The model under review builds one solid part; all positions refer to its coordinate system, in mm. A direction names the side the tool comes from. Round coordinates to 2 decimals unless told otherwise and drop trailing zeros. Order: outer loops, then holes, each group sorted by start corner. A loop starts at its lowest first (then second) coordinate and runs counter-clockwise, first axis right, second up. Notation, with made-up numbers: M 43,75 L 66,75 A11 ccw 66,86 Z; hole C 87,19.5 d6. An arc over 180 degrees is marked long. Answer as CSV lines item,"result". Start each with the question number.
from build123d import *

# Parameters (mm, degrees)
BOSS_EXTRUDE1_DEPTH = 12.7
SKETCH2_R           = 3.499999985
CUT_EXTRUDE1_DEPTH  = 127


with BuildPart() as part:
    # Sketch1 → Boss-Extrude1 (new body)
    with BuildSketch(Plane.XY):
        with BuildLine():
            Line((-3.110307402, -37.00399852), (-3.110307402, -54.746228005))
            Line((-3.110307402, -54.746228005), (-7.465236153, -54.746228005))
            Line((-7.465236153, -54.746228005), (-7.465236153, -42.046228005))
            ThreePointArc((-7.465236153, -42.046228005), (-12.933427118, -37.502447849), (-15.956082844, -31.067340787))
            ThreePointArc((-15.956082844, -31.067340787), (-18.522349701, -15.547297089), (-18.849139709, 0.180089543))
            ThreePointArc((-18.849139709, 0.180089543), (0, 18.85), (18.849139709, 0.180089543))
            ThreePointArc((18.849139709, 0.180089543), (18.522349701, -15.547297089), (15.956082844, -31.067340787))
            ThreePointArc((15.956082844, -31.067340787), (12.933427118, -37.502447849), (7.465236153, -42.046228005))
            Line((7.465236153, -42.046228005), (7.465236153, -54.746228005))
            Line((7.465236153, -54.746228005), (3.110307402, -54.746228005))
            Line((3.110307402, -54.746228005), (3.110307402, -37.00399852))
            ThreePointArc((3.110307402, -37.00399852), (7.417993382, -34.206219068), (9.768536138, -29.639088993))
            ThreePointArc((9.768536138, -29.639088993), (12.203438759, -14.918076577), (12.5, 0))
            ThreePointArc((12.5, 0), (0, 12.5), (-12.5, 0))
            ThreePointArc((-12.5, 0), (-12.203438759, -14.918076577), (-9.768536138, -29.639088993))
            ThreePointArc((-9.768536138, -29.639088993), (-7.417993382, -34.206219068), (-3.110307402, -37.00399852))
        make_face()
    extrude(amount=BOSS_EXTRUDE1_DEPTH)

    # Sketch2 → Cut-Extrude1 (cut)
    with BuildSketch(Plane(origin=(7.465236153, 0, 0), x_dir=(0, 0, -1), z_dir=(1, 0, 0))):
        with Locations(Location((-6.35, -48.396228005, 0), (0, 0, 90))):
            Circle(SKETCH2_R)
    extrude(amount=-CUT_EXTRUDE1_DEPTH, mode=Mode.SUBTRACT)


solid = part.part
Item 1: Tool access review of faces 1 (the flat face through (-7.465, -46, 3)), 2 (the cylindrical face through (0.275, 12.497, 6.261)), 3 (the flat face through (7.465, -45, 9)), 4 (the cylindrical face through (-5.257, -51.893, 6.504)), 5 (the flat face through (3.11, -44, 6)): name each direction out of +Z, -Z, +X, -X, +Y, -Y from which nothing blocks a thin tool from reaching the whole face with its end or side.
Item 2: Consider section B-B (y = -4.5). State the section outline as (x, z) points.
Item 3: For pin 1 (1 mm diameter, centred on y = 10, z = 4, fed in from +X); pin 2 (4 mm diameter, centred on y = -46, z = 3.5, fed in from -X); pin 3 (6.5 mm diameter, centred on y = -50, z = 5.5, fed in from +X); pin 4 (12 mm diameter, centred on x = -13.5, y = -32.5, fed in from -Z), all flat-tipped, find the tip position at first contact; note any pin that passes through.
Item 4: Wall thickness on probe 1 along X at (y, z) = (-5, 0.5); probe 2 along Y at (x, z) = (4, 8.25); probe 3 along Z at (x, y) = (7, -48.5): over which ranges is each line inside the solid? List them lowest first. Write a range as [from, to].
Item 5: The part is to be moulded in two halves that separate along X. For faces 6 (the flat face through (-5, -54.746, 6)), 7 (the cylindrical face through (18.542, -15.328, 6.261)), 8 (the cylindrical face through (12.184, -15.126, 6.261)), say which applies: +X half, -X half, draft (parallel to the pull), parting line (faces both ways), or undercut.
Item 6: Consider section D-D (x = -0.5). State the section outline as (y, z) points, and give its area (3 significant figures).
Reported:
1,face 1,"+Z, -Z, -X, -Y"
1,face 2,"+Z, -Z"
1,face 3,"+Z, -Z, +X, -Y"
1,face 4,"+X, -X"
1,face 5,"+Z, -Z, -Y"
2,outline,"M -18.99,0 L -12.64,0 L -12.64,12.7 L -18.99,12.7 Z; M 12.64,0 L 18.99,0 L 18.99,12.7 L 12.64,12.7 Z"
3,pin 1,"stops at x = 16.28"
3,pin 2,"stops at x = -7.47"
3,pin 3,"stops at x = 7.47"
3,pin 4,"stops at z = 0"
4,probe 1,"x = [-18.99, -12.64], [12.64, 18.99]"
4,probe 2,"y = [-54.75, -51.34], [-45.46, -36.67], [11.84, 18.42]"
4,probe 3,"z = [0, 2.85], [9.85, 12.7]"
5,face 6,"draft"
5,face 7,"+X half"
5,face 8,"undercut"
6,outline,"M 12.49,0 L 18.84,0 L 18.84,12.7 L 12.49,12.7 Z"
6,area,"80.7 mm²"
